Geometry check sheet. Reference: the model listing, model coordinates, mm. A direction names the side the tool comes from. Round coordinates to 2 decimals unless told otherwise and drop trailing zeros. Write each loop counter-clockwise with the first axis right and the second up, starting at its lowest first coordinate (ties: lowest second). Pieces come first, ordered by that corner, then holes. Notation, with made-up numbers: (0.25, 11.25) - (21.25, 11.25) arc R24 ccw to (21.25, 45.25) - close; hole circle Ø4 at (-19.75, 84). An arc over 180 degrees is marked (long way). Return JSON: item names as keys, results as strings.
```python
from build123d import *

# Parameters (mm, degrees)
F0_W     = 101.6
F0_H     = 101.6
F1_DEPTH = 25.4
F2_R     = 29.031913
F3_DEPTH = 25.4
F4_R     = 6.35
F5_DEPTH = 76.2
F6_R     = 10.005143
F7_DEPTH = 25.4


with BuildPart() as f1:
    # F0 (on Top) → F1 (new body)
    with BuildSketch(Plane.XY):
        Rectangle(F0_W, F0_H)
    extrude(amount=F1_DEPTH)

    # F2 (on face) → F3 (join)
    with BuildSketch(Plane.XY.offset(25.4)):
        Circle(F2_R)
    extrude(amount=F3_DEPTH)

    # F4 (on face) → F5 (join)
    with BuildSketch(Plane(origin=(0, 0, 0), x_dir=(1, 0, 0), z_dir=(0, 0, -1))):
        with Locations((-30.48, 30.48)):
            Circle(F4_R)
        with Locations((30.48, 30.48)):
            Circle(F4_R)
        with Locations((30.48, -30.48)):
            Circle(F4_R)
        with Locations((-30.48, -30.48)):
            Circle(F4_R)
    extrude(amount=F5_DEPTH)

    # F6 (on face) → F7 (join)
    with BuildSketch(Plane.XY.offset(50.8)):
        Circle(F6_R)
    extrude(amount=F7_DEPTH)


solid = f1.part
```
(1) Section check A-A, the plane y = 0. Enter the section's corners in (x, z).
Response values:
{"outline": "(-50.8, 0) - (50.8, 0) - (50.8, 25.4) - (29.03, 25.4) - (29.03, 50.8) - (10.01, 50.8) - (10.01, 76.2) - (-10.01, 76.2) - (-10.01, 50.8) - (-29.03, 50.8) - (-29.03, 25.4) - (-50.8, 25.4) - close"}
(2) Section check C-C, the plane z = 30.5. Enter the section's corners in (x, y), plus the area to 3 significant figures.
Response values:
{"outline": "circle Ø58.06 at (0, 0)", "area": "2,650 mm^2"}
(3) Material ranges on line 1 along X through (y, z) = (0.5, 50); line 2 along Z through (x, y) = (2.5, 14.5); line 3 along Z through (x, y) = (-12.5, 29), recorded low to high. Write a range as [from, to].
Response values:
{"line 1": "x = [-29.03, 29.03]", "line 2": "z = [0, 50.8]", "line 3": "z = [0, 25.4]"}
(4) Release check for a two-part mould opening along X. For faces 4 (the face through (-1, -50.8, 13)), 5 (the face through (-31.86, -24.28, -37.57)), 6 (the face through (-6.294, -28.342, 37.922)) record: pulls with the +X half, pulls with the -X half, needs draft (parallel to the pull), parting line crosses it, or undercut.
Response values:
{"face 4": "needs draft", "face 5": "undercut", "face 6": "parting line crosses it"}
(5) Access from +Z, -Z, +X, -X, +Y, -Y to the whole of each face (thin tool, end or side, straight path). Record for faces 1 (the face through (25.8, 26.19, -37.57)), 2 (the face through (30, 30, -76.2)), 3 (the face through (22, -22, 25.4)).
Response values:
{"face 1": "-Z", "face 2": "-Z, +X, -X, +Y, -Y", "face 3": "+Z"}
(6) Section check D-D, the plane y = -19. Enter the section's corners in (x, z), plus the area to 3 significant figures.
Response values:
{"outline": "(-50.8, 0) - (50.8, 0) - (50.8, 25.4) - (21.95, 25.4) - (21.95, 50.8) - (-21.95, 50.8) - (-21.95, 25.4) - (-50.8, 25.4) - close", "area": "3,700 mm^2"}
(7) Gauge pin test, flat ends, axial feed: pin 1 (4 mm diameter, centred on x = -28.5, z = -53, fed in from -Y); pin 2 (1 mm diameter, centred on x = 20, z = 53, fed in from -Y); pin 3 (17.5 mm diameter, centred on x = -7.5, y = 9, fed in from +Z); pin 4 (5 mm diameter, centred on x = 28, y = -2, fed in from -Z). Record the tip position at first contact, or that the pin passes through.
Response values:
{"pin 1": "stops at y = -36.83", "pin 2": "passes through", "pin 3": "stops at z = 76.2", "pin 4": "stops at z = 0"}
